Here's the drawing with two shaded views (mm, measured from the low corner). I have some questions. Round coordinates to 2 decimals unless told otherwise and drop trailing zeros. Loops run counter-clockwise (first coordinate to the right, second up) from the corner with the lowest first, then second, coordinate; pieces in that order, holes last. Notation, with made-up numbers: (54.25, -9.5) -> (99.25, -9.5) arc R19 cw to (99.25, 6.5) -> close; hole circle Ø7 at (47.5, 48.5). An arc over 180 degrees is marked (long way). Use a Markdown table: item, result.
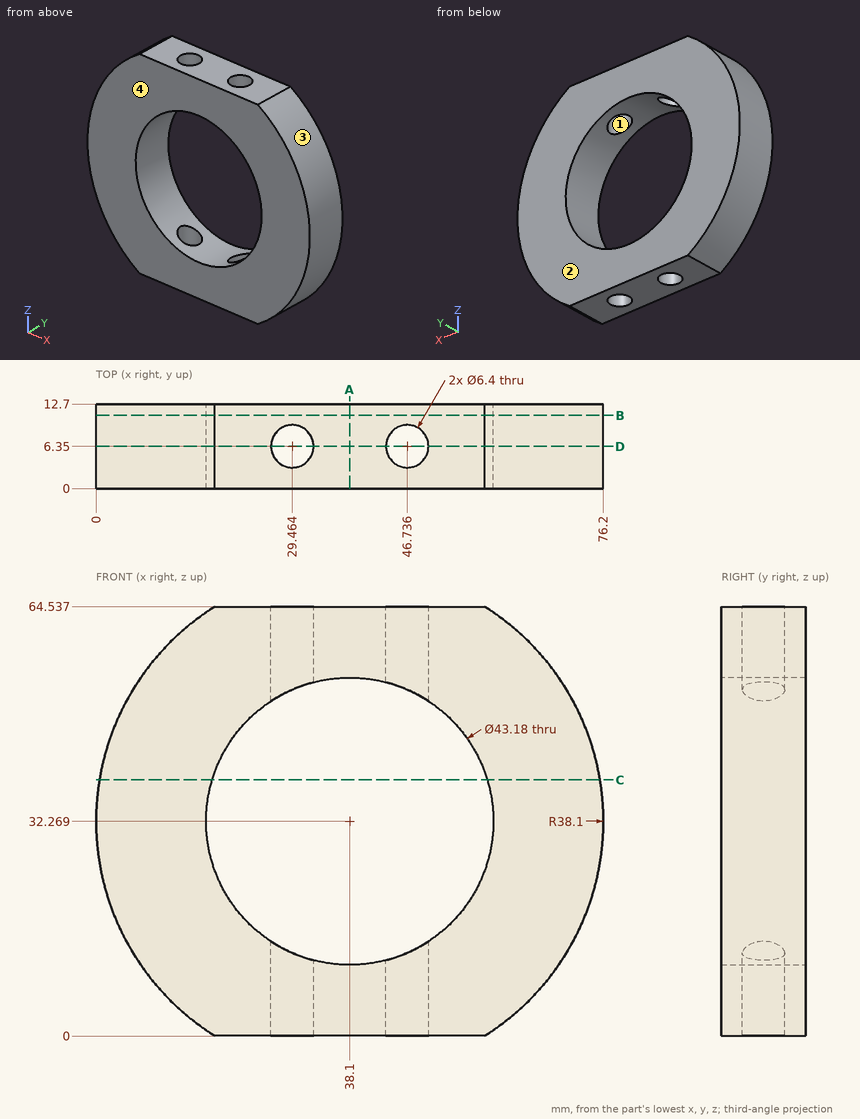
1. I need wall thicknesses on line 1 (Z direction, x = 37.5, y = 4.75); line 2 (X direction, y = 7.25, z = 10) (1 decimal); line 3 (Z direction, x = 42, y = 3.5). Which ranges of each line are inside material? Lowest first, please.
Answer sheet:
| item | result |
|---|---|
| line 1 | z = 0 to 10.69, 53.85 to 64.54 |
| line 2 | x = 7.2 to 26.4, 32.5 to 43.7, 49.8 to 69 |
| line 3 | z = 0 to 11.03, 53.5 to 64.54 |
2. If we mould it in two halves opening along Y, with no side actions, what happens to the marked faces 1, 2, 3 and 4? For each: +Y half, -Y half, draft (parallel to the pull), parting line (faces both ways), or undercut.
Answer sheet:
| item | result |
|---|---|
| face 1 | undercut |
| face 2 | +Y half |
| face 3 | draft |
| face 4 | -Y half |
3. I want a section at C-C (z = 38.5). Please give me the cut outline in (x, y), plus the area to 3 significant figures.
Answer sheet:
| item | result |
|---|---|
| outline | (0.51, 0) -> (17.43, 0) -> (17.43, 12.7) -> (0.51, 12.7) -> close; (58.77, 0) -> (75.69, 0) -> (75.69, 12.7) -> (58.77, 12.7) -> close |
| area | 430 mm² |
4. I want a section at A-A (x = 38.1). Please give me the cut outline in (y, z).
Answer sheet:
| item | result |
|---|---|
| outline | (0, 0) -> (12.7, 0) -> (12.7, 10.68) -> (0, 10.68) -> close; (0, 53.86) -> (12.7, 53.86) -> (12.7, 64.54) -> (0, 64.54) -> close |
5. I want a section at D-D (y = 6.35). Please give me the cut outline in (x, z) (1 decimal), plus the area to 3 significant figures.
Answer sheet:
| item | result |
|---|---|
| outline | (17.8, 0) -> (26.3, 0) -> (26.3, 14.2) arc R21.6 cw to (26.3, 50.3) -> (26.3, 64.5) -> (17.8, 64.5) arc R38.1 ccw to start; (32.7, 0) -> (43.5, 0) -> (43.5, 11.4) arc R21.6 cw to (32.7, 11.4) -> close; (32.7, 53.2) arc R21.6 cw to (43.5, 53.2) -> (43.5, 64.5) -> (32.7, 64.5) -> close; (49.9, 0) -> (58.4, 0) arc R38.1 ccw to (58.4, 64.5) -> (49.9, 64.5) -> (49.9, 50.3) arc R21.6 cw to (49.9, 14.2) -> close |
| area | 2,450 mm² |
6. I want a section at B-B (y = 11). Please give me the cut outline in (x, z).
Answer sheet:
| item | result |
|---|---|
| outline | (17.84, 0) -> (58.36, 0) arc R38.1 ccw to (58.36, 64.54) -> (17.84, 64.54) arc R38.1 ccw to start; hole circle Ø43.18 at (38.1, 32.27) |
7. Will these pins go through, and if not, where does the flat tip stop? pin 1 Ø1.5 at (x, y) = (60, 5.5) entering from +Z; pin 2 Ø1.5 at (y, z) = (9.5, 37.5) entering from +X (1 decimal).
Answer sheet:
| item | result |
|---|---|
| pin 1 | stops at z = 63.96 |
| pin 2 | stops at x = 75.9 |
